Model file for the job. Use its own axes, mm. Face numbers are marked on the shaded views. A direction names the side the tool comes from. Coordinates: 2 decimals unless noted, no trailing zeros. Loops run counter-clockwise (first coordinate to the right, second up) from the corner with the lowest first, then second, coordinate; pieces in that order, holes last.
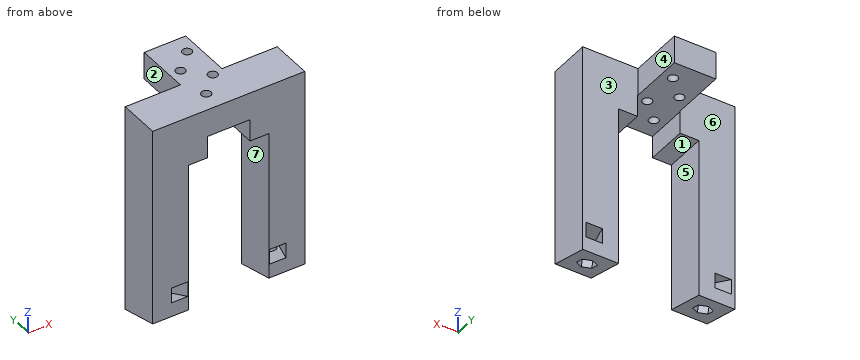
from build123d import *

# Parameters (mm, degrees)
BOSS_EXTRUDE1_DEPTH = 15
SKETCH2_W           = 15
SKETCH2_H           = 10
BOSS_EXTRUDE2_DEPTH = 19.8
CUT_EXTRUDE2_REACH  = 81.519
SKETCH4_R           = 1.7
LPATTERN1_COUNT     = 2
LPATTERN1_PITCH     = 14
CUT_EXTRUDE4_REACH  = 102.06
CUT_EXTRUDE5_START  = -38.811107067
CUT_EXTRUDE5_DEPTH  = 19.709275544
CUT_EXTRUDE6_DEPTH  = 3
CUT_EXTRUDE7_REACH  = 89.185
SKETCH10_R          = 1.85


# Read off the part's stored shape, not the designer's step: Cut-Extrude5
with BuildPart() as part:
    # Sketch1 → Boss-Extrude1 (new body)
    with BuildSketch(Plane(origin=(0, 0, 0), x_dir=(1, 0, 0), z_dir=(0, 1, 0))):
        Polygon((-27.5, 0), (27.5, 0), (27.5, 76), (14.5, 76), (14.5, 18), (7.7, 18), (7.7, 10), (-7.7, 10), (-7.7, 18), (-14.5, 18), (-14.5, 76), (-27.5, 76), align=None)
    extrude(amount=BOSS_EXTRUDE1_DEPTH)

    # Sketch2 → Boss-Extrude2 (add)
    with BuildSketch(Plane(origin=(0, 15, 0), x_dir=(1, 0, 0), z_dir=(0, 1, 0))):
        with Locations((0, 5)):
            Rectangle(SKETCH2_W, SKETCH2_H)
    extrude(amount=BOSS_EXTRUDE2_DEPTH)

    # Sketch4 → Cut-Extrude2 (cut, up to next)
    with BuildSketch(Plane(origin=(0, 0, -10), x_dir=(-1, 0, 0), z_dir=(0, 0, -1)), mode=Mode.PRIVATE) as cut_extrude2_sk1:
        with Locations((-3.5, 28)):
            Circle(SKETCH4_R)
    cut_extrude2_tool1 = extrude(cut_extrude2_sk1.sketch, amount=-CUT_EXTRUDE2_REACH, mode=Mode.PRIVATE) & part.part
    # Sketch4 → Cut-Extrude2 (cut, up to next)
    with BuildSketch(Plane(origin=(0, 0, -10), x_dir=(-1, 0, 0), z_dir=(0, 0, -1)), mode=Mode.PRIVATE) as cut_extrude2_sk2:
        with Locations((3.5, 21)):
            Circle(SKETCH4_R)
    cut_extrude2_tool2 = extrude(cut_extrude2_sk2.sketch, amount=-CUT_EXTRUDE2_REACH, mode=Mode.PRIVATE) & part.part
    cut_extrude2_1 = cut_extrude2_tool1.solids().sort_by_distance((3.5, 28, -10))[0]
    add(cut_extrude2_1, mode=Mode.SUBTRACT)
    cut_extrude2_2 = cut_extrude2_tool2.solids().sort_by_distance((-3.5, 21, -10))[0]
    add(cut_extrude2_2, mode=Mode.SUBTRACT)
    cut_extrude2 = cut_extrude2_1 + cut_extrude2_2  # Cut-Extrude2 as one shape, for the pattern or mirror that repeats it

    # LPattern1: Cut-Extrude2 ×2
    with Locations(*[(0, -i * LPATTERN1_PITCH, 0) for i in range(1, LPATTERN1_COUNT)]):
        add(cut_extrude2, mode=Mode.SUBTRACT)

    # Sketch7 → Cut-Extrude4 (cut, up to next)
    with BuildSketch(Plane.ZY.offset(27.5), mode=Mode.PRIVATE) as cut_extrude4_sk1:
        Polygon((-76, 15), (-72.25, 0), (-76, 0), align=None)
    cut_extrude4_tool1 = extrude(cut_extrude4_sk1.sketch, amount=-CUT_EXTRUDE4_REACH, mode=Mode.PRIVATE) & part.part
    cut_extrude4 = cut_extrude4_tool1.solids().sort_by_distance((-27.5, 5, -74.75))[0]
    add(cut_extrude4, mode=Mode.SUBTRACT)

    # Cut-Extrude5 outline → Cut-Extrude5 (cut)
    with BuildSketch(Plane(origin=(0, 0, 0), x_dir=(0.9396926207859096, 0.3318082769460259, -0.08295206923650612), z_dir=(0.34202014332566544, -0.9116357484973617, 0.2279089371243395)).offset(CUT_EXTRUDE5_START)):
        Polygon((-8.802397208, -59.757011885), (-14.302397208, -59.757011885), (-13.846160827, -65.092795636), (-8.346160827, -65.092795636), align=None)
    cut_extrude5 = extrude(amount=CUT_EXTRUDE5_DEPTH, mode=Mode.SUBTRACT)

    # Sketch9 → Cut-Extrude6 (cut)
    with BuildSketch(Plane(origin=(0, -17, -68), x_dir=(-1, 0, 0), z_dir=(0, -0.24253562503633286, -0.970142500145332))):
        Polygon((21, 22.054021957), (23.771281292, 23.654021957), (23.771281292, 26.854021957), (21, 28.454021957), (18.228718708, 26.854021957), (18.228718708, 23.654021957), align=None)
    cut_extrude6 = extrude(amount=-CUT_EXTRUDE6_DEPTH, mode=Mode.SUBTRACT)

    # Sketch10 → Cut-Extrude7 (cut, up to next)
    with BuildSketch(Plane(origin=(0, -16.272393125, -65.0895725), x_dir=(-1, 0, 0), z_dir=(0, -0.2425356250363299, -0.9701425001453328)), mode=Mode.PRIVATE) as cut_extrude7_sk1:
        with Locations(Location((21, 25.254021957, 0), (0, 0, 90))):
            Circle(SKETCH10_R)
    cut_extrude7_tool1 = extrude(cut_extrude7_sk1.sketch, amount=-CUT_EXTRUDE7_REACH, mode=Mode.PRIVATE) & part.part
    cut_extrude7 = cut_extrude7_tool1.solids().sort_by_distance((-21, 8.227607, -71.214572))[0]
    add(cut_extrude7, mode=Mode.SUBTRACT)

    # Mirror1: Cut-Extrude4, Cut-Extrude5, Cut-Extrude6, Cut-Extrude7 across plane
    add(cut_extrude4.mirror(Plane(origin=(0, 0, 0), x_dir=(0, 0, 1), z_dir=(1, 0, 0))), mode=Mode.SUBTRACT)
    add(cut_extrude5.mirror(Plane(origin=(0, 0, 0), x_dir=(0, 0, 1), z_dir=(1, 0, 0))), mode=Mode.SUBTRACT)
    add(cut_extrude6.mirror(Plane(origin=(0, 0, 0), x_dir=(0, 0, 1), z_dir=(1, 0, 0))), mode=Mode.SUBTRACT)
    add(cut_extrude7.mirror(Plane(origin=(0, 0, 0), x_dir=(0, 0, 1), z_dir=(1, 0, 0))), mode=Mode.SUBTRACT)


solid = part.part
Q1. Slice it at D-D (x = -3). List the corners of the cut face in (y, z), and give its area (3 significant figures).
Answers:
outline: (0, -10) - (5.38, -10) - (5.38, 0) - (0, 0) - close; (8.62, -10) - (19.38, -10) - (19.38, 0) - (8.62, 0) - close; (22.62, -10) - (34.8, -10) - (34.8, 0) - (22.62, 0) - close
area: 283 mm2
Q2. Slice it at C-C (y = 28). List the corners of the cut face in (x, z).
Answers:
outline: (-7.5, -10) - (1.8, -10) - (1.8, 0) - (-7.5, 0) - close; (5.2, -10) - (7.5, -10) - (7.5, 0) - (5.2, 0) - close
Q3. Drill centre lines: line 1 (Y direction, x = -3.5, z = -6.75); line 2 (Y direction, x = 3.5, z = -2.75); line 3 (Y direction, x = -15, z = -21). Where is each one in solid material? Low to high.
Answers:
line 1: y = 0 to 5.3, 8.7 to 19.3, 22.7 to 34.8
line 2: y = 0 to 12.3, 15.7 to 26.3, 29.7 to 34.8
line 3: y = 0 to 15
Q4. Which spindle directions (+Z, -Z, +X, -X, +Y, -Y) get a long thin tool onto all of the face, cutting with end or side? Do the marked faces 1, 2 and 3. Say none if no direction does.
Answers:
face 1: -Z, +Y, -Y
face 2: +Z, -Z, -X, +Y
face 3: +Z, -Z, +X, +Y
Q5. Mould opens along X. For the marked faces 4, 5, 6 and 7 say: +X half, -X half, draft (parallel to the pull), parting line (faces both ways), or undercut.
Answers:
face 4: +X half
face 5: undercut
face 6: draft
face 7: undercut
Q6. Slice it at A-A (z = -34). List the corners of the cut face in (x, y), and give its area (3 significant figures).
Answers:
outline: (-27.5, 0) - (-14.5, 0) - (-14.5, 15) - (-27.5, 15) - close; (14.5, 0) - (27.5, 0) - (27.5, 15) - (14.5, 15) - close
area: 390 mm2
Q7. Flat gauge pins, fed straight in: P1, Ø1.5, axis at x = 19.5, y = 5.5, coming from the -Z side; P2, Ø5.5, axis at x = -3.5, y = 21, coming from the +Z side; P3, Ø4.5, axis at x = 3.5, y = 28, coming from the -Z side; P4, Ø10, axis at x = -21.5, z = -33, coming from the +Y side. Where does each tip first touch, or does it go through?
Answers:
P1: stops at z = -73.66
P2: stops at z = 0
P3: stops at z = -10
P4: stops at y = 15
Q8. Slice it at B-B (y = 14). List the corners of the cut face in (x, z), and give its area (3 significant figures).
Answers:
outline: (-27.5, -75.75) - (-14.5, -75.75) - (-14.5, -18) - (-7.7, -18) - (-7.7, -10) - (1.8, -10) - (1.8, 0) - (-27.5, 0) - close; (5.2, -10) - (7.7, -10) - (7.7, -18) - (14.5, -18) - (14.5, -75.75) - (27.5, -75.75) - (27.5, 0) - (5.2, 0) - close; hole (-25.91, -70.6) - (-20.06, -70.6) - (-20.06, -65.1) - (-25.91, -65.1) - close; hole (20.06, -70.6) - (25.91, -70.6) - (25.91, -65.1) - (20.06, -65.1) - close
area: 2,270 mm2
